```python
from build123d import *

# Parameters (mm, degrees)
SKETCH_W      = 69.1
SKETCH_H      = 75.7
PAD_DEPTH     = 1.5
FILLET_R      = 5
SKETCH001_R   = 1.7
HOLE_DEPTH    = 25
SKETCH002_W   = 14
SKETCH002_H   = 14
SKETCH002_W_2 = 18.5
SKETCH002_H_2 = 9.5
POCKET_DEPTH  = 5
FILLET001_R   = 1


with BuildPart() as part:
    # Sketch → Pad (new body)
    with BuildSketch(Plane.XY):
        with Locations((34.55, 37.85)):
            Rectangle(SKETCH_W, SKETCH_H)
    extrude(amount=PAD_DEPTH)

    # Fillet
    fillet_edges = [part.edges().sort_by_distance(p)[0] for p in [
        (0, 0, 0.75),
        (69.1, 0, 0.75),
        (69.1, 75.7, 0.75),
        (0, 75.7, 0.75),
    ]]
    fillet(fillet_edges, radius=FILLET_R)

    # Sketch001 (on Face5 of Fillet) → Hole (cut)
    with BuildSketch(Plane.XY.offset(1.5)):
        with Locations((5, 5)):
            Circle(SKETCH001_R)
        with Locations((64.1, 5)):
            Circle(SKETCH001_R)
        with Locations((5, 70.7)):
            Circle(SKETCH001_R)
        with Locations((64.1, 70.7)):
            Circle(SKETCH001_R)
    extrude(amount=-HOLE_DEPTH, mode=Mode.SUBTRACT)

    # Sketch002 (on Face5 of Hole) → Pocket (cut)
    with BuildSketch(Plane.XY.offset(1.5)):
        with Locations((26.2, 26.2)):
            Rectangle(SKETCH002_W, SKETCH002_H)
        with Locations((45.2, 26.2)):
            Rectangle(SKETCH002_W, SKETCH002_H)
        with Locations((26.2, 45.2)):
            Rectangle(SKETCH002_W, SKETCH002_H)
        with Locations((45.2, 45.2)):
            Rectangle(SKETCH002_W, SKETCH002_H)
        with Locations((34.25, 70.95)):
            Rectangle(SKETCH002_W_2, SKETCH002_H_2)
    extrude(amount=-POCKET_DEPTH, mode=Mode.SUBTRACT)

    # Fillet001
    fillet001_edges = [part.edges().sort_by_distance(p)[0] for p in [
        (19.2, 52.2, 0.75),
        (38.2, 52.2, 0.75),
        (38.2, 33.2, 0.75),
        (19.2, 33.2, 0.75),
        (38.2, 38.2, 0.75),
        (38.2, 19.2, 0.75),
        (19.2, 19.2, 0.75),
        (52.2, 19.2, 0.75),
        (33.2, 19.2, 0.75),
        (19.2, 38.2, 0.75),
        (52.2, 52.2, 0.75),
        (52.2, 33.2, 0.75),
        (33.2, 33.2, 0.75),
        (33.2, 52.2, 0.75),
    ]]
    fillet(fillet001_edges, radius=FILLET001_R)


solid = part.part
```
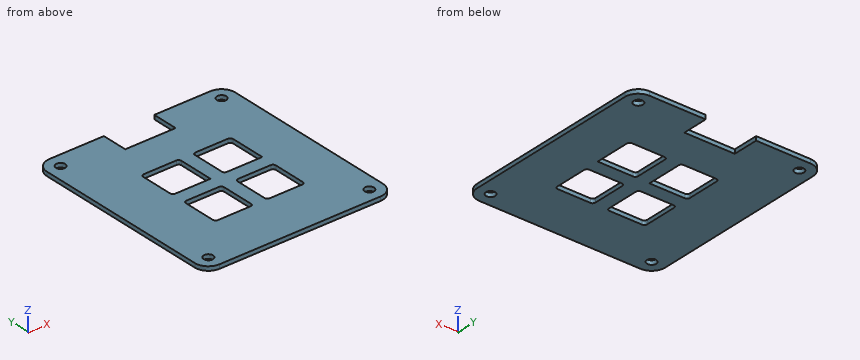
Source: CAD feature listing. Evaluate the final solid. Frame: model axes, mm. Round coordinates to 2 decimals unless told otherwise and drop trailing zeros. Order: outer loops, then holes, each group sorted by start corner. A loop starts at its lowest first (then second) coordinate and runs counter-clockwise, first axis right, second up. Notation, with made-up numbers: (-35.75, -39) -> (8.25, -39) arc R20 ccw to (8.25, -10) -> close; hole circle Ø11 at (-37.5, -30). An arc over 180 degrees is marked (long way). One line per item, written item: value. Start each with the question number.
Q1. Section query A-A (y = 67.5). Return the cut outline in (x, z), plus the area to 3 significant figures.
Q2. Material intervals for probe 1 along Y at (x, z) = (64.1, 0.9); probe 2 along X at (y, z) = (70.5, 1.25); probe 3 along X at (y, z) = (27, 0.15), sorted ascending.
Q3. Section query B-B (z = 0.7). Give the number of separate pieces and of enclosed holes in the cut face, plus the area to 3 significant figures.
Findings below:
1. outline: (0, 0) -> (25, 0) -> (25, 1.5) -> (0, 1.5) -> close; (43.5, 0) -> (69.1, 0) -> (69.1, 1.5) -> (43.5, 1.5) -> close
1. area: 75.9 mm²
2. probe 1: 0 to 3.3, 6.7 to 69, 72.4 to 75.7
2. probe 2: 0 to 3.31, 6.69 to 25, 43.5 to 62.41, 65.79 to 69.1
2. probe 3: 0 to 19.2, 33.2 to 38.2, 52.2 to 69.1
3. separate pieces: 1
3. enclosed holes: 8
3. area: 4,220 mm²
